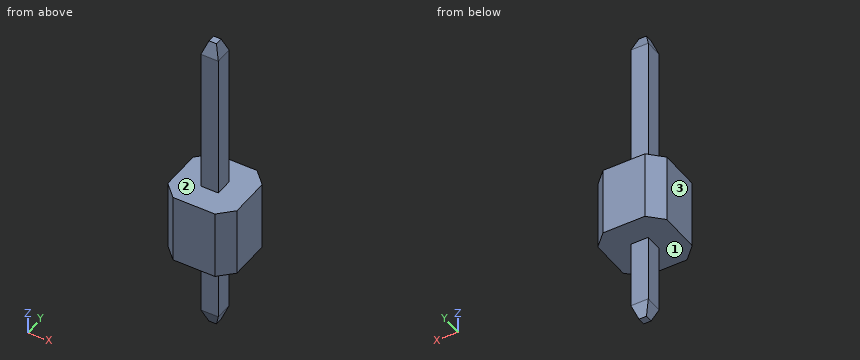
```python
from build123d import *

# Parameters (mm, degrees)
SKETCH1_W             = 0.64
SKETCH1_H             = 0.64
BOSS_EXTRUDE1_DEPTH   = 8.4
SKETCH2_W             = 0.64
SKETCH2_H             = 0.64
BOSS_EXTRUDE2_DEPTH   = 3
CHAMFER1_SIZE         = 0.5
CHAMFER1_SIZE2        = 0.181985117
CHAMFER1_PART_2_SIZE  = 0.5
CHAMFER1_PART_2_SIZE2 = 0.181985117
CHAMFER1_PART_3_SIZE  = 0.5
CHAMFER1_PART_3_SIZE2 = 0.181985117
CHAMFER1_PART_4_SIZE  = 0.5
CHAMFER1_PART_4_SIZE2 = 0.181985117
SKETCH3_W             = 2.54
SKETCH3_H             = 2.5
BOSS_EXTRUDE3_DEPTH   = 2.54
CHAMFER2_SIZE         = 0.5


with BuildPart() as part:
    # Sketch1 → Boss-Extrude1 (new body)
    with BuildSketch(Plane.XY):
        Rectangle(SKETCH1_W, SKETCH1_H)
    extrude(amount=BOSS_EXTRUDE1_DEPTH)

    # Sketch2 → Boss-Extrude2 (add)
    with BuildSketch(Plane(origin=(0, 0, 0), x_dir=(-1, 0, 0), z_dir=(0, 0, -1))):
        Rectangle(SKETCH2_W, SKETCH2_H)
    extrude(amount=BOSS_EXTRUDE2_DEPTH)

    # Chamfer1
    chamfer1_edges = [part.edges().sort_by_distance(p)[0] for p in [
        (0.32, 0, 8.4),
        (0.32, 0, -3),
    ]]
    chamfer1_side = [part.faces().sort_by_distance(p)[0] for p in [
        (0.32, 0, 2.7),
    ]]
    chamfer(chamfer1_edges, length=CHAMFER1_SIZE, length2=CHAMFER1_SIZE2, reference=chamfer1_side[0])

    # Chamfer1 part 2
    chamfer1_part_2_edges = [part.edges().sort_by_distance(p)[0] for p in [
        (0, 0.32, 8.4),
        (0, 0.32, -3),
    ]]
    chamfer1_part_2_side = [part.faces().sort_by_distance(p)[0] for p in [
        (0, 0.32, 2.7),
    ]]
    chamfer(chamfer1_part_2_edges, length=CHAMFER1_PART_2_SIZE, length2=CHAMFER1_PART_2_SIZE2, reference=chamfer1_part_2_side[0])

    # Chamfer1 part 3
    chamfer1_part_3_edges = [part.edges().sort_by_distance(p)[0] for p in [
        (-0.32, 0, -3),
        (-0.32, 0, 8.4),
    ]]
    chamfer1_part_3_side = [part.faces().sort_by_distance(p)[0] for p in [
        (-0.32, 0, 2.7),
    ]]
    chamfer(chamfer1_part_3_edges, length=CHAMFER1_PART_3_SIZE, length2=CHAMFER1_PART_3_SIZE2, reference=chamfer1_part_3_side[0])

    # Chamfer1 part 4
    chamfer1_part_4_edges = [part.edges().sort_by_distance(p)[0] for p in [
        (0, -0.32, -3),
        (0, -0.32, 8.4),
    ]]
    chamfer1_part_4_side = [part.faces().sort_by_distance(p)[0] for p in [
        (0, -0.32, 2.7),
    ]]
    chamfer(chamfer1_part_4_edges, length=CHAMFER1_PART_4_SIZE, length2=CHAMFER1_PART_4_SIZE2, reference=chamfer1_part_4_side[0])

    # Sketch3 → Boss-Extrude3 (add)
    with BuildSketch(Plane.XY):
        Rectangle(SKETCH3_W, SKETCH3_H)
    extrude(amount=BOSS_EXTRUDE3_DEPTH)

    # Chamfer2
    chamfer2_edges = [part.edges().sort_by_distance(p)[0] for p in [
        (-1.27, 1.25, 1.27),
        (-1.27, -1.25, 1.27),
        (1.27, -1.25, 1.27),
        (1.27, 1.25, 1.27),
    ]]
    chamfer(chamfer2_edges, length=CHAMFER2_SIZE)


solid = part.part
```
Here's how the part is built. I have some questions about the finished solid (model axes, mm). Face numbers are marked on the shaded views. A direction names the side the tool comes from. Coordinates: 2 decimals unless noted, no trailing zeros. Order: outer loops, then holes, each group sorted by start corner. A loop starts at its lowest first (then second) coordinate and runs counter-clockwise, first axis right, second up.
Item 1: If we section it at B-B, the plane x = 0: List the corners of the cut face in (y, z) for me.
Response values:
outline: (-1.25, 0) - (-0.32, 0) - (-0.32, -2.5) - (-0.14, -3) - (0.14, -3) - (0.32, -2.5) - (0.32, 0) - (1.25, 0) - (1.25, 2.54) - (0.32, 2.54) - (0.32, 7.9) - (0.14, 8.4) - (-0.14, 8.4) - (-0.32, 7.9) - (-0.32, 2.54) - (-1.25, 2.54) - close
Item 2: If we section it at C-C, the plane y = 0.85: List the corners of the cut face in (x, z) for me.
Response values:
outline: (-1.17, 0) - (1.17, 0) - (1.17, 2.54) - (-1.17, 2.54) - close
Item 3: If we section it at A-A, the plane z = 1.25: List the corners of the cut face in (x, y) for me.
Response values:
outline: (-1.27, -0.75) - (-0.77, -1.25) - (0.77, -1.25) - (1.27, -0.75) - (1.27, 0.75) - (0.77, 1.25) - (-0.77, 1.25) - (-1.27, 0.75) - close
Item 4: I need wall thicknesses on probe 1 along Z at (x, y) = (-0.8, 0.1); probe 2 along X at (y, z) = (0.15, 5.5). Which ranges of each line are inside material? Lowest first, please.
Response values:
probe 1: z = 0 to 2.54
probe 2: x = -0.32 to 0.32
Item 5: Which directions (+Z, -Z, +X, -X, +Y, -Y) give clear straight access to the entire face, cutting with the end or side of a thin tool? Please do the marked faces 1, 2 and 3.
Response values:
face 1: -Z
face 2: +Z
face 3: +Z, -Z, -X, +Y, -Y
Item 6: I'm going to push flat-ended pins straight in: pin 1 Ø1 at (y, z) = (0.5, 4.5) entering from -X; pin 2 Ø0.7 at (y, z) = (0, -2) entering from +X; pin 3 Ø0.7 at (x, z) = (0, 5.5) entering from -Y. Where does each tip first touch, or does it pass through?
Response values:
pin 1: stops at x = -0.32
pin 2: stops at x = 0.32
pin 3: stops at y = -0.32
Item 7: If we section it at D-D, the plane x = 0.6: List the corners of the cut face in (y, z) for me, then the cut area to 3 significant figures.
Response values:
outline: (-1.25, 0) - (1.25, 0) - (1.25, 2.54) - (-1.25, 2.54) - close
area: 6.35 mm2
